Autodesk Inventor part; units mm, degrees
ref_plane "YZ Plane" through (0, 0, 0) normal (1, 0, 0) x (0, 1, 0)
ref_plane "XZ Plane" through (0, 0, 0) normal (0, 1, 0) x (-1, 0, 0)
ref_plane "XY Plane" through (0, 0, 0) normal (0, 0, 1) x (1, 0, 0)
sketch "Skizze1" plane through (0, 0, 0) normal (0, 1, 0) x (-1, 0, 0)
  line L0 (0, 0) -> (3.35, 0)
  line L1 (3.35, 0) -> (3.35, -8)
  line L2 (3.35, -8) -> (4.85, -8)
  line L3 (4.85, -8) -> (4.85, -9.4)
  line L4 (4.85, -9.4) -> (3.35, -9.4)
  line L5 (3.35, -9.4) -> (3.35, -15.7)
  line L6 (3.35, -15.7) -> (1.5, -15.7)
  line L7 (1.5, -15.7) -> (1.5, -19.2)
  line L8 (1.5, -19.2) -> (3.35, -19.2)
  line L9 (3.35, -19.2) -> (3.35, -21.2)
  line L10 (3.35, -21.2) -> (0, -21.2)
  line L11 (0, 0) -> (0, -21.2)
  dimension "d0" = 3.35
  dimension "d1" = 8
  dimension "d3" = 5.5
  dimension "d4" = 11.8
  dimension "d5" = 21.2
  dimension "d6" = 2
  dimension "d7" = 1.5
  dimension "d10" = 4.85
revolve "Umdrehung1" add sketch "Skizze1" angle 360 about axis through (0, 0, 0) along (0, 0, -1)
properties part number "licht_taster"
Geometry check sheet. Reference: the model listing, model coordinates, mm. A direction names the side the tool comes from. Round coordinates to 2 decimals unless told otherwise and drop trailing zeros. Order: outer loops, then holes, each group sorted by start corner. A loop starts at its lowest first (then second) coordinate and runs counter-clockwise, first axis right, second up. Notation, with made-up numbers: (-18, 20) - (20, 20) arc R35 ccw to (20, 57) - close; hole circle Ø2 at (81.25, 83). An arc over 180 degrees is marked (long way). Use a Markdown table: item, result. Add a question column.
1) Mould release check, pull along Y, two halves, no side actions. Record for faces 1 (the cylindrical face through (1.5, 0.07, -17.47)), 2 (the flat face through (2, 0, -15.7)): released by +Y, released by -Y, zero draft, split by the parting line, or undercut.
2) Section check C-C (x = -1.75). Record the cut outline in (y, z).
3) Set-up check for faces 3 (the cylindrical face through (3.347, 0.147, -4.056)), 4 (the cylindrical face through (3.347, 0.147, -12.594)), 5 (the flat face through (2, 0, -19.2)): record each of +Z, -Z, +X, -X, +Y, -Y from which the full face is reachable in a straight line by a thin tool's end or side.
4) Section check B-B (x = 0). Record the cut outline in (y, z), then the cut area to 3 significant figures.
5) Gauge pin test, flat ends, axial feed: P1, Ø5, axis at x = 2, z = -13.5, coming from the -Y side; P2, Ø1.5, axis at x = 2.5, z = -15.5, coming from the -Y side; P3, Ø2, axis at x = -1.5, z = -18, coming from the +Y side. Record the tip position at first contact, or that the pin passes through.
6) Thickness scan on line 1 along Z through (x, y) = (1.25, -2); line 2 along Z through (x, y) = (-3, -2); line 3 along Y through (x, z) = (0, -16). Record the ranges inside material, lowest first.
7) Section check A-A (y = -2.75). Record the cut outline in (x, z) (3 decimals), then the cut area to 3 significant figures.
Established:
| question | item | result |
|---|---|---|
| 1 | face 1 | split by the parting line |
| 1 | face 2 | zero draft |
| 2 | outline | (-4.52, -9.4) - (-2.86, -9.4) - (-2.86, -15.7) - (2.86, -15.7) - (2.86, -9.4) - (4.52, -9.4) - (4.52, -8) - (2.86, -8) - (2.86, 0) - (-2.86, 0) - (-2.86, -8) - (-4.52, -8) - close; (-2.86, -21.2) - (2.86, -21.2) - (2.86, -19.2) - (-2.86, -19.2) - close |
| 3 | face 3 | +Z |
| 3 | face 4 | -Z |
| 3 | face 5 | none |
| 4 | outline | (-4.85, -9.4) - (-3.35, -9.4) - (-3.35, -15.7) - (-1.5, -15.7) - (-1.5, -19.2) - (-3.35, -19.2) - (-3.35, -21.2) - (3.35, -21.2) - (3.35, -19.2) - (1.5, -19.2) - (1.5, -15.7) - (3.35, -15.7) - (3.35, -9.4) - (4.85, -9.4) - (4.85, -8) - (3.35, -8) - (3.35, 0) - (-3.35, 0) - (-3.35, -8) - (-4.85, -8) - close |
| 4 | area | 133 mm2 |
| 5 | P1 | y = -3.35 |
| 5 | P2 | y = -2.86 |
| 5 | P3 | y = 1.41 |
| 6 | line 1 | -21.2 to -19.2, -15.7 to 0 |
| 6 | line 2 | -9.4 to -8 |
| 6 | line 3 | -1.5 to 1.5 |
| 7 | outline | (-3.995, -9.4) - (-1.913, -9.4) - (-1.913, -15.7) - (1.913, -15.7) - (1.913, -9.4) - (3.995, -9.4) - (3.995, -8) - (1.913, -8) - (1.913, 0) - (-1.913, 0) - (-1.913, -8) - (-3.995, -8) - close; (-1.913, -21.2) - (1.913, -21.2) - (1.913, -19.2) - (-1.913, -19.2) - close |
| 7 | area | 73.6 mm2 |
